```python
from build123d import *

# Parameters (mm, degrees)
ESBO_O1_R                = 1.5
RESSALTO_EXTRUS_O1_DEPTH = 1.6


with BuildPart() as part:
    # Esboço1 → Ressalto-extrusão1 (new body)
    with BuildSketch(Plane(origin=(0, 0, 0), x_dir=(1, 0, 0), z_dir=(0, 1, 0))):
        with BuildLine():
            ThreePointArc((-52.484604611, -22.234349076), (-50.025216279, 0), (-52.484604611, 22.234349076))
            ThreePointArc((-52.484604611, 22.234349076), (-55.425625842, 32), (-45.497813442, 34.335826363))
            ThreePointArc((-45.497813442, 34.335826363), (-25.01260814, 43.323108128), (-6.98679117, 56.570175439))
            ThreePointArc((-6.98679117, 56.570175439), (0, 64), (6.98679117, 56.570175439))
            ThreePointArc((6.98679117, 56.570175439), (25.01260814, 43.323108128), (45.497813442, 34.335826363))
            ThreePointArc((45.497813442, 34.335826363), (55.425625842, 32), (52.484604611, 22.234349076))
            ThreePointArc((52.484604611, 22.234349076), (50.025216279, 0), (52.484604611, -22.234349076))
            ThreePointArc((52.484604611, -22.234349076), (55.425625842, -32), (45.497813442, -34.335826363))
            ThreePointArc((45.497813442, -34.335826363), (25.01260814, -43.323108128), (6.98679117, -56.570175439))
            ThreePointArc((6.98679117, -56.570175439), (0, -64), (-6.98679117, -56.570175439))
            ThreePointArc((-6.98679117, -56.570175439), (-25.01260814, -43.323108128), (-45.497813442, -34.335826363))
            ThreePointArc((-45.497813442, -34.335826363), (-55.425625842, -32), (-52.484604611, -22.234349076))
        make_face()
        with Locations(Location((-49.363448016, 28.5, 0), (0, 0, 270))):
            Circle(ESBO_O1_R, mode=Mode.SUBTRACT)
        with Locations(Location((-49.363448016, -28.5, 0), (0, 0, 270))):
            Circle(ESBO_O1_R, mode=Mode.SUBTRACT)
        with Locations(Location((0, -57, 0), (0, 0, 270))):
            Circle(ESBO_O1_R, mode=Mode.SUBTRACT)
        with Locations(Location((49.363448016, -28.5, 0), (0, 0, 270))):
            Circle(ESBO_O1_R, mode=Mode.SUBTRACT)
        with Locations(Location((49.363448016, 28.5, 0), (0, 0, 270))):
            Circle(ESBO_O1_R, mode=Mode.SUBTRACT)
        with Locations(Location((0, 57, 0), (0, 0, 270))):
            Circle(ESBO_O1_R, mode=Mode.SUBTRACT)
    extrude(amount=RESSALTO_EXTRUS_O1_DEPTH)


solid = part.part
```
Source: CAD feature listing. Evaluate the final solid. Frame: model axes, mm. Give positions to 0.01 mm unless a question says otherwise; leave off trailing zeros. Loops run counter-clockwise (first coordinate to the right, second up) from the corner with the lowest first, then second, coordinate; pieces in that order, holes last. Notation, with made-up numbers: M -37.75,-7.5 L 3.25,-7.5 A23 ccw 3.25,25.5 Z; hole C 51,3.25 d3. An arc over 180 degrees is marked long. Put each result on its own line as item: value.
Q1. Pin query (flat end, axial travel): P1, Ø2.5, axis at x = -49.36, z = 28.5, coming from the +Y side. Return the tip coordinate at first contact, or that it passes through.
Response values:
P1: passes through
Q2. Section C-C (x = -41.5). Return the cut outline in (y, z).
Response values:
outline: M 0,-35.68 L 1.6,-35.68 L 1.6,35.68 L 0,35.68 Z
Q3. Section D-D (z = -42). Return the cut outline in (x, y).
Response values:
outline: M -27.38,0 L 27.38,0 L 27.38,1.6 L -27.38,1.6 Z
Q4. Section B-B (y = 0.5). Return the cut outline in (x, z), and give its area (3 significant figures).
Response values:
outline: M -52.48,-22.23 A7 ccw long -45.5,-34.34 A101.74 cw -6.99,-56.57 A7 ccw long 6.99,-56.57 A101.74 cw 45.5,-34.34 A7 ccw long 52.48,-22.23 A101.74 cw 52.48,22.23 A7 ccw long 45.5,34.34 A101.74 cw 6.99,56.57 A7 ccw long -6.99,56.57 A101.74 cw -45.5,34.34 A7 ccw long -52.48,22.23 A101.74 cw Z; hole C -49.36,-28.5 d3; hole C -49.36,28.5 d3; hole C 0,-57 d3; hole C 0,57 d3; hole C 49.36,-28.5 d3; hole C 49.36,28.5 d3
area: 9,390 mm²
Q5. Line query: probe 1 along X at (y, z) = (0.65, 28.5); probe 2 along X at (y, z) = (0.6, -28); probe 3 along X at (y, z) = (1.1, 57). Output: solid intervals per line, ascending. Write a range as [from, to].
Response values:
probe 1: x = [-56.36, -50.86], [-47.86, 47.86], [50.86, 56.36]
probe 2: x = [-56.35, -50.78], [-47.95, 47.95], [50.78, 56.35]
probe 3: x = [-7, -1.5], [1.5, 7]
Q6. Section A-A (z = -28.5). Return the cut outline in (x, y), and give its area (3 significant figures).
Response values:
outline: M -56.36,0 L -50.86,0 L -50.86,1.6 L -56.36,1.6 Z; M -47.86,0 L 47.86,0 L 47.86,1.6 L -47.86,1.6 Z; M 50.86,0 L 56.36,0 L 56.36,1.6 L 50.86,1.6 Z
area: 171 mm²
